```python
from build123d import *

# Parameters (mm, degrees)
SKETCH1_W                  = 46
SKETCH1_H                  = 27
SKETCH1_R                  = 3.75
BOSS_EXTRUDE1_DEPTH        = 2
SKETCH7_W                  = 3.5
SKETCH7_H                  = 27
BOSS_EXTRUDE4_DEPTH        = 8
CUT_EXTRUDE3_REACH         = 47.305
SKETCH8_W                  = 19.5
SKETCH8_H                  = 8
CUT_EXTRUDE4_REACH         = 38.541
CUT_EXTRUDE5_REACH         = 39.03
SKETCH10_R                 = 0.75
CHAMFER1_SIZE              = 1
LPATTERN1_COUNT            = 2
LPATTERN1_PITCH            = 4
CHAMFER1_OF_LPATTERN1_SIZE = 1


# Read off the part's stored shape, not the designer's step: Mirror2
with BuildPart() as part:
    # Sketch1 → Boss-Extrude1 (new body)
    with BuildSketch(Plane(origin=(0, 0, 0), x_dir=(1, 0, 0), z_dir=(0, 1, 0))):
        with Locations((10, 0)):
            Rectangle(SKETCH1_W, SKETCH1_H)
        with Locations(Location((0, 0, 0), (0, 0, 270))):
            Circle(SKETCH1_R, mode=Mode.SUBTRACT)
    extrude(amount=BOSS_EXTRUDE1_DEPTH)

    # Sketch7 → Boss-Extrude4 (add)
    with BuildSketch(Plane.XZ):
        with Locations((31.25, 0)):
            Rectangle(SKETCH7_W, SKETCH7_H)
    extrude(amount=BOSS_EXTRUDE4_DEPTH)

    # Sketch8 → Cut-Extrude3 (cut, up to next)
    with BuildSketch(Plane.ZY.offset(-29.5), mode=Mode.PRIVATE) as cut_extrude3_sk1:
        with Locations((0, -4)):
            Rectangle(SKETCH8_W, SKETCH8_H)
    cut_extrude3_tool1 = extrude(cut_extrude3_sk1.sketch, amount=-CUT_EXTRUDE3_REACH, mode=Mode.PRIVATE) & part.part
    add(cut_extrude3_tool1.solids().sort_by_distance((29.5, -4, 0))[0], mode=Mode.SUBTRACT)

    # Sketch9 → Cut-Extrude4 (cut, up to next)
    with BuildSketch(Plane.XZ, mode=Mode.PRIVATE) as cut_extrude4_sk1:
        with BuildLine():
            Line((-9, 11.7), (26.5, 11.7))
            ThreePointArc((26.5, 11.7), (28.2, 10), (26.5, 8.3))
            Line((26.5, 8.3), (-9, 8.3))
            ThreePointArc((-9, 8.3), (-10.7, 10), (-9, 11.7))
        make_face()
    cut_extrude4_tool1 = extrude(cut_extrude4_sk1.sketch, amount=-CUT_EXTRUDE4_REACH, mode=Mode.PRIVATE) & part.part
    cut_extrude4 = cut_extrude4_tool1.solids().sort_by_distance((8.75, 0, 10))[0]
    add(cut_extrude4, mode=Mode.SUBTRACT)

    # Mirror1: Cut-Extrude4 across plane
    add(cut_extrude4.mirror(Plane.XY), mode=Mode.SUBTRACT)

    # Sketch10 → Cut-Extrude5 (cut, up to next)
    with BuildSketch(Plane(origin=(0, 2, 0), x_dir=(1, 0, 0), z_dir=(0, 1, 0)), mode=Mode.PRIVATE) as cut_extrude5_sk1:
        with Locations(Location((-6.5, 0, 0), (0, 0, 270))):
            Circle(SKETCH10_R)
    cut_extrude5_tool1 = extrude(cut_extrude5_sk1.sketch, amount=-CUT_EXTRUDE5_REACH, mode=Mode.PRIVATE) & part.part
    cut_extrude5 = cut_extrude5_tool1.solids().sort_by_distance((-6.5, 2, 0))[0]
    add(cut_extrude5, mode=Mode.SUBTRACT)

    # Chamfer1
    chamfer1_edges = [part.edges().sort_by_distance(p)[0] for p in [
        (-6.5, 0, -0.75),
    ]]
    chamfer(chamfer1_edges, length=CHAMFER1_SIZE)

    # LPattern1: Cut-Extrude5 ×2
    with Locations(*[(-i * LPATTERN1_PITCH, 0, 0) for i in range(1, LPATTERN1_COUNT)]):
        add(cut_extrude5, mode=Mode.SUBTRACT)

    # Chamfer1 of LPattern1
    chamfer1_of_lpattern1_edges = [part.edges().sort_by_distance(p)[0] for p in [
        (-10.5, 0, -0.75),
    ]]
    chamfer(chamfer1_of_lpattern1_edges, length=CHAMFER1_OF_LPATTERN1_SIZE)

    # Mirror2 outline → Mirror2 (revolve, cut)
    with BuildSketch(Plane(origin=(6.5, 0, 0), x_dir=(1, 0, 0), z_dir=(0, 0, 1))):
        Polygon((0, 0), (1.75, 0), (0.75, 1), (0.75, 2), (0, 2), align=None)
    revolve(axis=Axis((6.5, 0, 0), (0, 1, 0)), mode=Mode.SUBTRACT)

    # Mirror2 2 outline → Mirror2 2 (revolve, cut)
    with BuildSketch(Plane(origin=(10.5, 0, 0), x_dir=(1, 0, 0), z_dir=(0, 0, 1))):
        Polygon((0, 0), (1.75, 0), (0.75, 1), (0.75, 2), (0, 2), align=None)
    revolve(axis=Axis((10.5, 0, 0), (0, 1, 0)), mode=Mode.SUBTRACT)


solid = part.part
```
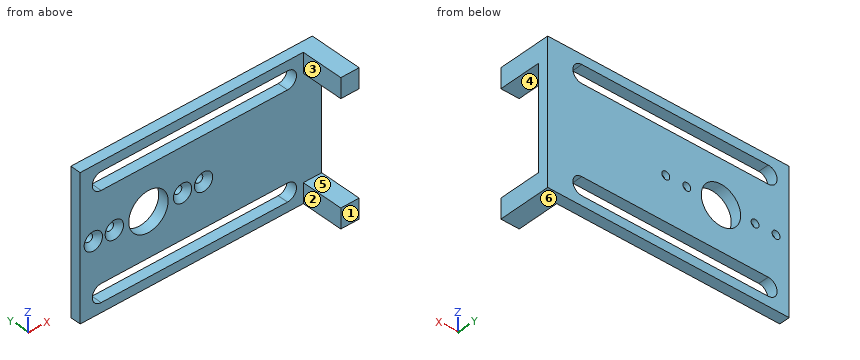
The listing builds one solid part. Answer for the finished solid, in the listing's coordinates (mm). Face numbers are marked on the shaded views. A direction names the side the tool comes from. Give positions to 0.01 mm unless a question says otherwise; leave off trailing zeros. Loops run counter-clockwise (first coordinate to the right, second up) from the corner with the lowest first, then second, coordinate; pieces in that order, holes last. Notation, with made-up numbers: (9.5, 85) - (19.5, 85) arc R26 cw to (19.5, 117) - close; hole circle Ø2 at (1.25, 61). An arc over 180 degrees is marked (long way). Answer as CSV lines item,"result". Start each with the question number.
Item 1: Find the intervals of material crossed by line 1 (Z direction, x = 20.5, y = 0.5); line 2 (X direction, y = 1.4, z = 0); line 3 (Z direction, x = 10.5, y = 1.7), in increasing order. Write a range as from..to.
Item 2: A cutting plane is placed at B-B on z = 0. Count the separate pieces of the cut face and the enclosed holes in it, then the cut area to 3 significant figures.
Item 3: For the marked faces 1 and 2, determine the directions among +Z, -Z, +X, -X, +Y, -Y from which every point of the face is accessible in a straight line to the end or side of a thin tool.
Item 4: A cutting plane is placed at D-D on x = -6.5. Determine the outline of the cut face in (y, z), then the cut area to 3 significant figures.
Item 5: Each of these flat-tipped pins is pushed along its axis until it touches: pin 1 (10 mm diameter, centred on x = 10.5, z = -10, fed in from +Y); pin 2 (2.5 mm diameter, centred on x = 6.5, z = 0, fed in from -Y); pin 3 (10 mm diameter, centred on x = 3.5, z = -10, fed in from -Y); pin 4 (1.9 mm diameter, centred on y = -4.5, z = 12, fed in from -X). Where does it stop, or does it pass through?
Item 6: A cutting plane is placed at A-A on y = -6.5. Determine the outline of the cut face in (x, z), then the cut area to 4 significant figures.
Item 7: A cutting plane is placed at C-C on x = 3. Determine the outline of the cut face in (y, z).
Item 8: The mould has two halves that part along Z. Classify the marked faces 3, 4, 5 and 6: +Z half, -Z half, draft (parallel to the pull), parting line (faces both ways), or undercut.
Found:
1,line 1,"z = -13.5..-11.7, -8.3..8.3, 11.7..13.5"
1,line 2,"x = -13..-11.25, -9.75..-7.25, -5.75..-3.75, 3.75..5.75, 7.25..9.75, 11.25..33"
1,line 3,"z = -13.5..-11.7, -8.3..-0.75, 0.75..8.3, 11.7..13.5"
2,separate pieces,"6"
2,enclosed holes,"0"
2,area,"61.0 mm^2"
3,face 1,"+Z, -Z, +X, -X, -Y"
3,face 2,"+Z, -Z, -X, -Y"
4,outline,"(0, -13.5) - (2, -13.5) - (2, -11.7) - (0, -11.7) - close; (0, -8.3) - (2, -8.3) - (2, -0.75) - (1, -0.75) - (0, -1.75) - close; (0, 1.75) - (1, 0.75) - (2, 0.75) - (2, 8.3) - (0, 8.3) - close; (0, 11.7) - (2, 11.7) - (2, 13.5) - (0, 13.5) - close"
4,area,"36.4 mm^2"
5,pin 1,"stops at y = 2"
5,pin 2,"stops at y = 0.5"
5,pin 3,"stops at y = 0"
5,pin 4,"stops at x = 29.5"
6,outline,"(29.5, -13.5) - (33, -13.5) - (33, -9.75) - (29.5, -9.75) - close; (29.5, 9.75) - (33, 9.75) - (33, 13.5) - (29.5, 13.5) - close"
6,area,"26.25 mm^2"
7,outline,"(0, -13.5) - (2, -13.5) - (2, -11.7) - (0, -11.7) - close; (0, -8.3) - (2, -8.3) - (2, -2.25) - (0, -2.25) - close; (0, 2.25) - (2, 2.25) - (2, 8.3) - (0, 8.3) - close; (0, 11.7) - (2, 11.7) - (2, 13.5) - (0, 13.5) - close"
8,face 3,"draft"
8,face 4,"undercut"
8,face 5,"undercut"
8,face 6,"-Z half"
